Job drawing, mm, ordinate dimensions from the low corner. One solid piece. Give positions to 0.01 mm unless a question says otherwise; leave off trailing zeros. Order: outer loops, then holes, each group sorted by start corner. A loop starts at its lowest first (then second) coordinate and runs counter-clockwise, first axis right, second up. Notation, with made-up numbers: (-35, -8) -> (19, -8) arc R10 ccw to (19, 9) -> close; hole circle Ø11 at (87, 78). An arc over 180 degrees is marked (long way). Write item = value, one per line. Start each with the question number.
(1) Saw through at C-C, the plane x = 315. List the corners of the cut face in (y, z).
(2) Probe line 1 along X through (y, z) = (562, 86.5); line 2 along Y through (x, z) = (704, 108). List the from-to ranges inside material, lowest first. Write a range as from..to.
(3) Saw through at B-B, the plane z = 305.5. List the corners of the cut face in (x, y), then the cut area to 3 significant figures.
(4) Flat gauge pin, fed straight in: pin 1 (12 mm diameter, centred on x = 1162.5, z = 530, fed in from -Y). Where does the tip first touch, or does it go through?
(5) Saw through at A-A, the plane y = 568.5. List the corners of the cut face in (x, z), then the cut area to 3 significant figures.
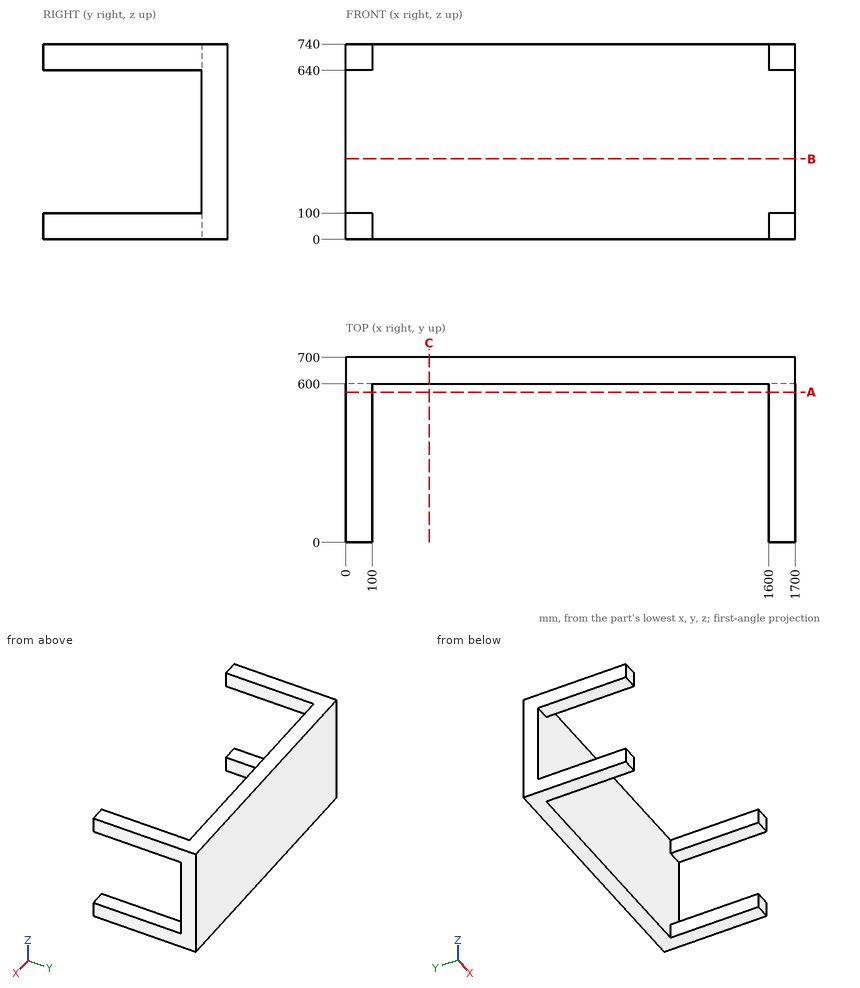
Results list:
q1.outline = (600, 0) -> (700, 0) -> (700, 740) -> (600, 740) -> close
q2.line_1 = 0..100, 1600..1700
q2.line_2 = 600..700
q3.outline = (0, 600) -> (1700, 600) -> (1700, 700) -> (0, 700) -> close
q3.area = 170,000 mm^2
q4.pin_1 = 600
q5.outline = (0, 0) -> (100, 0) -> (100, 100) -> (0, 100) -> close; (0, 640) -> (100, 640) -> (100, 740) -> (0, 740) -> close; (1600, 0) -> (1700, 0) -> (1700, 100) -> (1600, 100) -> close; (1600, 640) -> (1700, 640) -> (1700, 740) -> (1600, 740) -> close
q5.area = 40,000 mm^2
